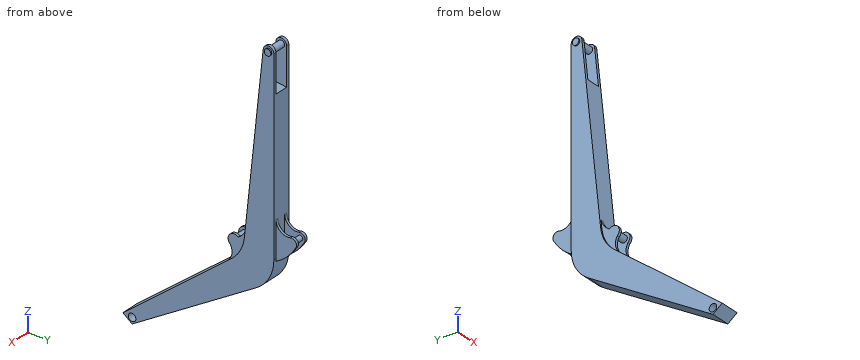
from build123d import *

# Parameters (mm, degrees)
SKETCH1_R           = 31
BOSS_EXTRUDE1_DEPTH = 77.5
CUT_EXTRUDE1_DEPTH  = 55
SKETCH3_R           = 27
BOSS_EXTRUDE2_DEPTH = 87.5
BOSS_EXTRUDE3_START = 55
SKETCH4_R           = 20
BOSS_EXTRUDE3_DEPTH = 20
BOSS_EXTRUDE4_START = 65
SKETCH5_R           = 28
BOSS_EXTRUDE4_DEPTH = 20
SKETCH6_R           = 20
BOSS_EXTRUDE5_DEPTH = 55
SKETCH7_R           = 28
BOSS_EXTRUDE6_DEPTH = 65


with BuildPart() as part:
    # Sketch1 → Boss-Extrude1 (new, symmetric)
    with BuildSketch(Plane(origin=(0, 0, 0), x_dir=(0, 0, -1), z_dir=(1, 0, 0))):
        with BuildLine():
            Line((-1649, 128.575159042), (-100.623018779, 128.575159042))
            ThreePointArc((-100.623018779, 128.575159042), (47.370818148, 90.689624097), (158.95669611, -13.646761532))
            Line((158.95669611, -13.646761532), (813.901849353, -1039.177258296))
            Line((813.901849353, -1039.177258296), (757.478946429, -1115.606676884))
            Line((757.478946429, -1115.606676884), (18.502038696, -221.191618301))
            ThreePointArc((18.502038696, -221.191618301), (-70.923814933, -147.926895035), (-181.413689889, -113.916742069))
            Line((-181.413689889, -113.916742069), (-1653.599252384, 40.816195646))
            ThreePointArc((-1653.599252384, 40.816195646), (-1692.939699529, 86.877941117), (-1649, 128.575159042))
        make_face()
        with Locations((764, -1039.424840958)):
            Circle(SKETCH1_R, mode=Mode.SUBTRACT)
    extrude(amount=BOSS_EXTRUDE1_DEPTH, both=True)

    # Sketch2 → Cut-Extrude1 (cut, symmetric)
    with BuildSketch(Plane(origin=(0, 0, 0), x_dir=(0, 0, -1), z_dir=(1, 0, 0))):
        with BuildLine():
            Line((-1337.780808047, 128.575159042), (-1350.221049377, 8.929861623))
            Line((-1350.221049377, 8.929861623), (-1653.599252384, 40.816195646))
            ThreePointArc((-1653.599252384, 40.816195646), (-1692.939699529, 86.877941117), (-1649, 128.575159042))
            Line((-1649, 128.575159042), (-1337.780808047, 128.575159042))
        make_face()
    extrude(amount=CUT_EXTRUDE1_DEPTH, both=True, mode=Mode.SUBTRACT)

    # Sketch3 → Boss-Extrude2 (add, symmetric)
    with BuildSketch(Plane(origin=(0, 0, 0), x_dir=(0, 0, -1), z_dir=(1, 0, 0))):
        with Locations((-1649, 84.575159042)):
            Circle(SKETCH3_R)
    extrude(amount=BOSS_EXTRUDE2_DEPTH, both=True)

    # Sketch4 → Boss-Extrude3 (add)
    with BuildSketch(Plane(origin=(0, 0, 0), x_dir=(0, 0, -1), z_dir=(1, 0, 0)).offset(BOSS_EXTRUDE3_START)):
        with BuildLine():
            Line((-100.623018779, 128.575159042), (-393.648383075, 128.575159042))
            ThreePointArc((-393.648383075, 128.575159042), (-318.488676572, 165.471643499), (-301.710632022, 247.501084968))
            ThreePointArc((-301.710632022, 247.501084968), (-287.401961188, 289.269705737), (-243.363225881, 292.423359888))
            ThreePointArc((-243.363225881, 292.423359888), (-150.511724148, 221.544648068), (-80.648383075, 127.926771904))
            ThreePointArc((-80.648383075, 127.926771904), (-90.630440565, 128.41301958), (-100.623018779, 128.575159042))
        make_face()
        with Locations((-263, 257.575159042)):
            Circle(SKETCH4_R, mode=Mode.SUBTRACT)
    extrude(amount=-BOSS_EXTRUDE3_DEPTH)

    # Mirror1: part across plane


with BuildPart() as part_1:
    add(part.part)
    add(part.part.mirror(Plane(origin=(0, 0, 0), x_dir=(0, 0, 1), z_dir=(1, 0, 0))))

    # Sketch5 → Boss-Extrude4 (add)
    with BuildSketch(Plane(origin=(0, 0, 0), x_dir=(0, 0, -1), z_dir=(1, 0, 0)).offset(BOSS_EXTRUDE4_START)):
        with BuildLine():
            Line((18.502038696, -221.191618301), (49.264592926, -258.424840958))
            ThreePointArc((49.264592926, -258.424840958), (-11.948195085, -227.059459611), (-79.255928514, -241.217905281))
            ThreePointArc((-79.255928514, -241.217905281), (-149.793064323, -246.168912443), (-154.744071486, -175.631776635))
            ThreePointArc((-154.744071486, -175.631776635), (-194.614118429, -131.834300288), (-248.329147356, -106.883644085))
            Line((-248.329147356, -106.883644085), (-181.413689889, -113.916742069))
            ThreePointArc((-181.413689889, -113.916742069), (-70.923814933, -147.926895035), (18.502038696, -221.191618301))
        make_face()
        with Locations((-117, -208.424840958)):
            Circle(SKETCH5_R, mode=Mode.SUBTRACT)
    extrude(amount=-BOSS_EXTRUDE4_DEPTH)

    # Mirror2: part across plane


with BuildPart() as part_2:
    add(part_1.part)
    add(part_1.part.mirror(Plane(origin=(0, 0, 0), x_dir=(0, 0, 1), z_dir=(1, 0, 0))))

    # Sketch6 → Boss-Extrude5 (add, symmetric)
    with BuildSketch(Plane(origin=(0, 0, 0), x_dir=(0, 0, -1), z_dir=(1, 0, 0))):
        with Locations((-263, 257.575159042)):
            Circle(SKETCH6_R)
    extrude(amount=BOSS_EXTRUDE5_DEPTH, both=True)

    # Sketch7 → Boss-Extrude6 (add, symmetric)
    with BuildSketch(Plane(origin=(0, 0, 0), x_dir=(0, 0, -1), z_dir=(1, 0, 0))):
        with Locations(Location((-117, -208.424840958, 0), (0, 0, 180))):
            Circle(SKETCH7_R)
    extrude(amount=BOSS_EXTRUDE6_DEPTH, both=True)


solid = part_2.part
Here's how the part is built. I have some questions about the finished solid (model axes, mm). Coordinates: 2 decimals unless noted, no trailing zeros. Write each loop counter-clockwise with the first axis right and the second up, starting at its lowest first coordinate (ties: lowest second). Pieces come first, ordered by that corner, then holes.
1) If we section it at D-D (y = -938.5): List the corners of the cut face in (x, z) for me, plus the area to 3 significant figures.
Filled in:
outline: (-77.5, -749.61) - (77.5, -749.61) - (77.5, -611.15) - (-77.5, -611.15) - close
area: 21,500 mm2
2) If we section it at B-B (y = -142): List the corners of the cut face in (x, z) for me, plus the area to 3 significant figures.
Filled in:
outline: (-77.5, -240.93) - (77.5, -240.93) - (77.5, 82.57) - (65, 82.57) - (65, 182.22) - (45, 182.22) - (45, 82.57) - (-45, 82.57) - (-45, 182.22) - (-65, 182.22) - (-65, 82.57) - (-77.5, 82.57) - close
area: 54,100 mm2
3) If we section it at C-C (z = 810): List the corners of the cut face in (x, y) for me.
Filled in:
outline: (-77.5, -47.85) - (77.5, -47.85) - (77.5, 128.58) - (-77.5, 128.58) - close
4) If I drill on line 1 (Y direction, x = 15, z = -764); line 2 (X direction, y = -107, z = -204); line 3 (Y direction, x = 17.5, z = 738), over which ranges is the centre line in solid material (lowest first)?
Filled in:
line 1: y = -1106.77 to -1070.42, -1008.42 to -961.04
line 2: x = -77.5 to 77.5
line 3: y = -55.42 to 128.58
5) I'm going to push flat-ended pins straight in: pin 1 (12 mm diameter, centred on x = 64.5, y = -219, fed in from -Z); pin 2 (3 mm diameter, centred on x = -27.5, z = -385.5, fed in from +Y); pin 3 (6 mm diameter, centred on x = 57.5, y = -337, fed in from -Z). Where does each tip first touch, or does it pass through?
Filled in:
pin 1: stops at z = -293.94
pin 2: stops at y = -366.03
pin 3: stops at z = -367.38
6) If we section it at A-A (z = 1451): List the corners of the cut face in (x, y) for me.
Filled in:
outline: (-77.5, 19.52) - (-55, 19.52) - (-55, 128.58) - (-77.5, 128.58) - close; (55, 19.52) - (77.5, 19.52) - (77.5, 128.58) - (55, 128.58) - close
